Can you work these out from the drawing? Everything is in mm from the part's minimum corner. Give positions to 0.01 mm unless a question says otherwise; leave off trailing zeros. Write each loop counter-clockwise with the first axis right and the second up, starting at its lowest first coordinate (ties: lowest second). Pieces come first, ordered by that corner, then holes. Notation, with made-up numbers: (25.25, -2.75) - (58.25, -2.75) arc R26 ccw to (58.25, 19.25) - close; hole circle Ø9 at (56, 85). An arc over 180 degrees is marked (long way). Write each question's results on one line, items separated by ' | '. Start each with the question number.
Item 1: Will these pins go through, and if not, where does the flat tip stop? P1, Ø1, axis at x = 33, z = 24.5, coming from the -Y side; P2, Ø4, axis at y = 7, z = 59.5, coming from the +X side; P3, Ø6, axis at x = 30.5, z = 21.5, coming from the -Y side; P4, Ø3, axis at y = 3.5, z = 81.5, coming from the +X side.
Item 2: Suppose I cut it at B-B on x = 8. List the corners of the cut face in (y, z) for me, then the cut area to 3 significant figures.
Item 3: Suppose I cut it at C-C on y = 5. List the corners of the cut face in (x, z) for me.
Item 4: Suppose I cut it at A-A on z = 80. List the corners of the cut face in (x, y) for me, then the cut area to 3 significant figures.
Item 5: Please list where these lines run through material, in increasing order: line 1 along Y through (x, z) = (6, 80); line 2 along Y through (x, z) = (14, 37.5); line 3 along X through (y, z) = (3.5, 77).
Item 6: Suppose I cut it at D-D on x = 34. List the corners of the cut face in (y, z) for me, then the cut area to 3 significant figures.
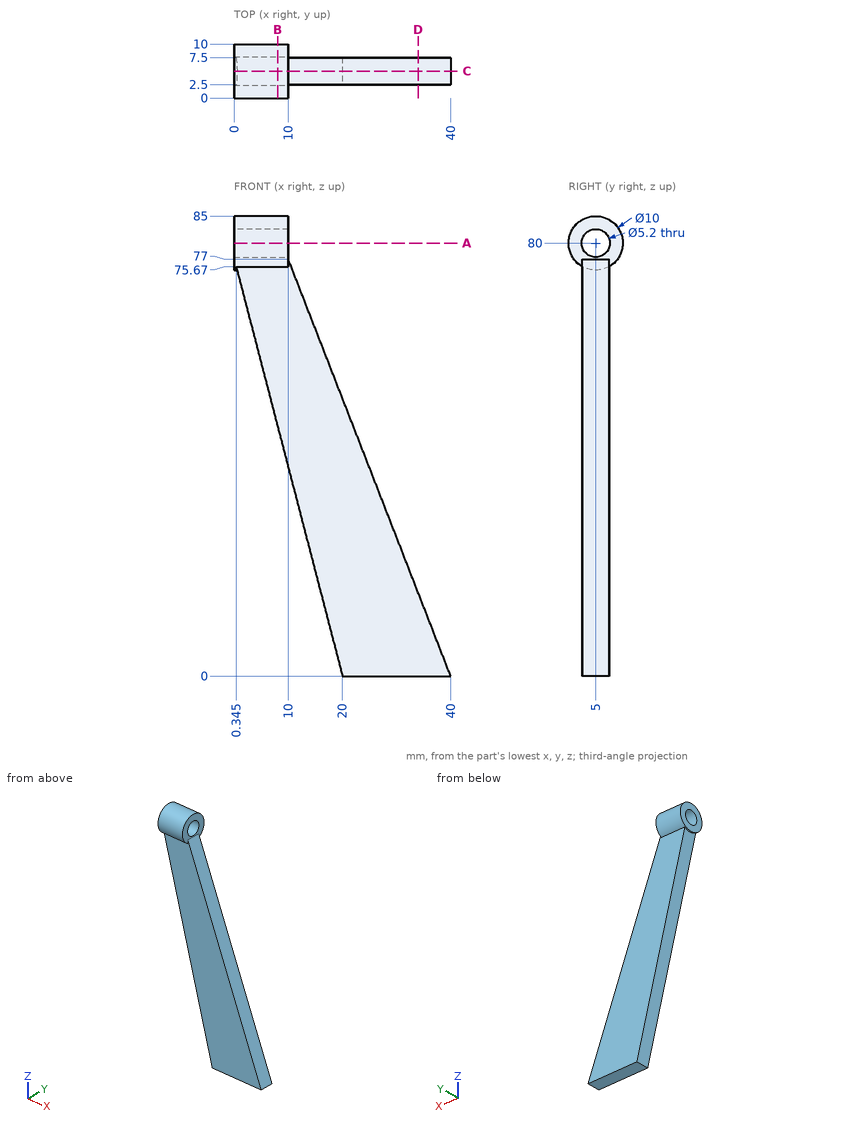
Checked values:
1) P1: passes through | P2: stops at x = 17.6 | P3: stops at y = 2.5 | P4: stops at x = 10
2) outline: (2.5, 46.2) - (7.5, 46.2) - (7.5, 75.67) arc R5 ccw (long way) to (2.5, 75.67) - close; hole circle Ø5.2 at (5, 80) | area: 202 mm^2
3) outline: (0, 75) - (0.52, 75) - (20, 0) - (40, 0) - (10, 77) - (10, 77.4) - (0, 77.4) - close; (0, 82.6) - (10, 82.6) - (10, 85) - (0, 85) - close
4) outline: (0, 0) - (10, 0) - (10, 2.4) - (0, 2.4) - close; (0, 7.6) - (10, 7.6) - (10, 10) - (0, 10) - close | area: 48.0 mm^2
5) line 1: y = 0 to 2.4, 7.6 to 10 | line 2: y = 2.5 to 7.5 | line 3: x = 0 to 10
6) outline: (2.5, 0) - (7.5, 0) - (7.5, 15.4) - (2.5, 15.4) - close | area: 77.0 mm^2
